from build123d import *

# Parameters (mm, degrees)
SKETCH_1_R          = 41
SKETCH_1_R_2        = 39
EXTRUDE_1_DEPTH     = 30
SKETCH_2_R          = 39
SKETCH_2_R_2        = 37
EXTRUDE_2_DEPTH     = 24
EXTRUDE_3_OUTLINE_R = 37
EXTRUDE_3_DEPTH     = 3
SKETCH_5_R          = 1.45
EXTRUDE_4_DEPTH     = 23
SKETCH_6_R          = 1.45
EXTRUDE_5_DEPTH     = 25
SKETCH_7_R          = 3.022472912
EXTRUDE_6_DEPTH     = 20
SKETCH_8_R          = 1.45
EXTRUDE_7_DEPTH     = 27
SKETCH_9_R          = 3.022472912
EXTRUDE_8_DEPTH     = 22


# Read off the part's stored shape, not the designer's step: the extrude step
with BuildPart() as part:
    # Sketch 1 → Extrude 1 (new body)
    with BuildSketch(Plane.XY):
        Circle(SKETCH_1_R)
        Circle(SKETCH_1_R_2, mode=Mode.SUBTRACT)
    extrude(amount=EXTRUDE_1_DEPTH)

    # Sketch 2 → Extrude 2 (add)
    with BuildSketch(Plane.XY):
        Circle(SKETCH_2_R)
        Circle(SKETCH_2_R_2, mode=Mode.SUBTRACT)
    extrude(amount=EXTRUDE_2_DEPTH)

    # Extrude 3 outline → Extrude 3 (add)
    with BuildSketch(Plane.XY):
        Circle(EXTRUDE_3_OUTLINE_R)
    extrude(amount=EXTRUDE_3_DEPTH)

    # Sketch 5 → Extrude 4 (add)
    with BuildSketch(Plane.XY.offset(3)):
        with Locations((-1.382493562, -21)):
            Circle(SKETCH_5_R)
    extrude(amount=EXTRUDE_4_DEPTH)

    # Sketch 6 → Extrude 5 (add)
    with BuildSketch(Plane.XY.offset(3)):
        with Locations((15.732786494, -10.652672394)):
            Circle(SKETCH_6_R)
    extrude(amount=EXTRUDE_5_DEPTH)

    # Sketch 7 → Extrude 6 (add)
    with BuildSketch(Plane.XY.offset(3)):
        with Locations((15.732786494, -10.652672394)):
            Circle(SKETCH_7_R)
    extrude(amount=EXTRUDE_6_DEPTH)

    # Sketch 8 → Extrude 7 (add)
    with BuildSketch(Plane.XY.offset(3)):
        with Locations((17, 9.307141481)):
            Circle(SKETCH_8_R)
    extrude(amount=EXTRUDE_7_DEPTH)

    # Sketch 9 → Extrude 8 (add)
    with BuildSketch(Plane.XY.offset(3)):
        with Locations((17, 9.307141481)):
            Circle(SKETCH_9_R)
    extrude(amount=EXTRUDE_8_DEPTH)


solid = part.part
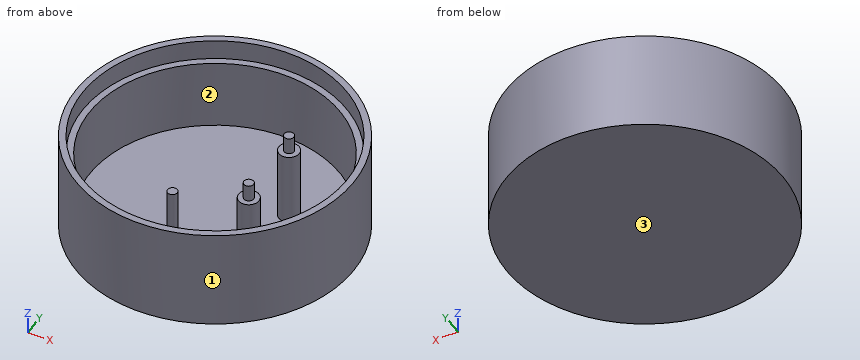
The model under review builds one solid part; all positions refer to its coordinate system, in mm. Face numbers are marked on the shaded views. Round coordinates to 2 decimals unless told otherwise and drop trailing zeros. Loops run counter-clockwise (first coordinate to the right, second up) from the corner with the lowest first, then second, coordinate; pieces in that order, holes last. Notation, with made-up numbers: (80, -20.5) -> (125, -20.5) arc R18 cw to (125, 6.5) -> close; hole circle Ø6 at (-36, 74.5). An arc over 180 degrees is marked (long way). Return JSON: item names as keys, results as strings.
(1) Add section D-D on y = -21. Write out the cut boundary in (x, z).
Solved:
{"outline": "(-35.21, 0) -> (35.21, 0) -> (35.21, 30) -> (32.86, 30) -> (32.86, 24) -> (30.46, 24) -> (30.46, 3) -> (0.07, 3) -> (0.07, 26) -> (-2.83, 26) -> (-2.83, 3) -> (-30.46, 3) -> (-30.46, 24) -> (-32.86, 24) -> (-32.86, 30) -> (-35.21, 30) -> close"}
(2) For line 1 (X direction, y = 8.5, z = 16.5); line 2 (Y direction, x = -1, z = 14); line 3 (Z direction, x = -6, y = -19.5), list the stretches that pass through material, from the lowest coordinate up.
Solved:
{"line 1": "-40.11 to -36.01, 14.09 to 19.91, 36.01 to 40.11", "line 2": "-40.99 to -36.99, -22.4 to -19.6, 36.99 to 40.99", "line 3": "0 to 3"}
(3) Add section C-C on x = 27. Write out the cut boundary in (y, z), plus the area to 3 significant figures.
Solved:
{"outline": "(-30.85, 0) -> (30.85, 0) -> (30.85, 30) -> (28.14, 30) -> (28.14, 24) -> (25.3, 24) -> (25.3, 3) -> (-25.3, 3) -> (-25.3, 24) -> (-28.14, 24) -> (-28.14, 30) -> (-30.85, 30) -> close", "area": "451 mm2"}
(4) Add section B-B on y = 0. Write out the cut boundary in (x, z).
Solved:
{"outline": "(-41, 0) -> (41, 0) -> (41, 30) -> (39, 30) -> (39, 24) -> (37, 24) -> (37, 3) -> (-37, 3) -> (-37, 24) -> (-39, 24) -> (-39, 30) -> (-41, 30) -> close"}
(5) The part is to be moulded in two halves that separate along X. For the marked faces 1, 2 and 3, say which applies: released by +X, released by -X, zero draft, split by the parting line, or undercut.
Solved:
{"face 1": "split by the parting line", "face 2": "undercut", "face 3": "zero draft"}
(6) Add section A-A on z = 7.75. Write out the cut boundary in (x, y).
Solved:
{"outline": "circle Ø82 at (0, 0); circle Ø2.9 at (-1.38, -21); circle Ø6.04 at (15.73, -10.65); circle Ø6.04 at (17, 9.31); hole circle Ø74 at (0, 0)"}
(7) For pin 1 (1 mm diameter, centred on x = 14.5, z = 24.5, fed in from -Y); pin 2 (1.4 mm diameter, centred on x = -1.5, y = -21, fed in from +Z); pin 3 (8 mm diameter, centred on y = -24, z = 13.5, fed in from -X), all flat-tipped, find the tip position at first contact; note any pin that passes through.
Solved:
{"pin 1": "y = -38.54", "pin 2": "z = 26", "pin 3": "x = -35.79"}
